Job drawing, mm, ordinate dimensions from the low corner. One solid piece. Coordinates: 2 decimals unless noted, no trailing zeros. Order: outer loops, then holes, each group sorted by start corner. A loop starts at its lowest first (then second) coordinate and runs counter-clockwise, first axis right, second up. Notation, with made-up numbers: M 56.25,-20.75 L 82.25,-20.75 A26 ccw 82.25,8.25 Z; hole C -38.75,54 d3. An arc over 180 degrees is marked long. Write item = value, one per line. Start each with the question number.
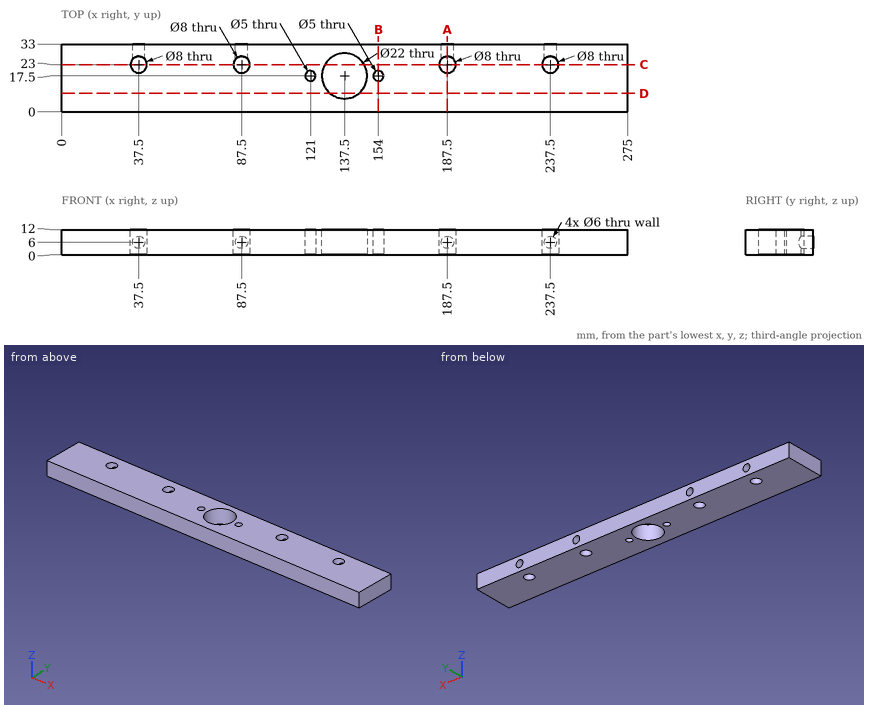
1. Flat gauge pin, fed straight in: pin 1 (5 mm diameter, centred on x = 87.5, z = 6, fed in from +Y). Where does the tip first touch, or does it go through?
2. Slice it at A-A (x = 187.5). Write the cut outline in (y, z).
3. Slice it at C-C (y = 23). Write the cut outline in (x, z).
4. Probe L1, parallel to X at y = 29.75, z = 6; L2, parallel to Y at x = 138.5, z = 1; L3, parallel to Z at x = 38, y = 30. List the from-to ranges inside material, lowest first.
5. Slice it at B-B (x = 154). Write the cut outline in (y, z), plus the area to 3 significant figures.
6. Slice it at D-D (y = 9). Write the cut outline in (x, z).
Calculated:
q1.pin_1 = 19.88
q2.outline = M 0,0 L 19,0 L 19,12 L 0,12 Z; M 27,0 L 33,0 L 33,3 L 27,3 Z; M 27,9 L 33,9 L 33,12 L 27,12 Z
q3.outline = M 0,0 L 33.5,0 L 33.5,12 L 0,12 Z; M 41.5,0 L 83.5,0 L 83.5,12 L 41.5,12 Z; M 91.5,0 L 127.97,0 L 127.97,12 L 91.5,12 Z; M 147.03,0 L 183.5,0 L 183.5,12 L 147.03,12 Z; M 191.5,0 L 233.5,0 L 233.5,12 L 191.5,12 Z; M 241.5,0 L 275,0 L 275,12 L 241.5,12 Z
q4.L1 = 0 to 34.5, 40.5 to 84.5, 90.5 to 184.5, 190.5 to 234.5, 240.5 to 275
q4.L2 = 0 to 6.55, 28.45 to 33
q4.L3 = 0 to 3.04, 8.96 to 12
q5.outline = M 0,0 L 15,0 L 15,12 L 0,12 Z; M 20,0 L 33,0 L 33,12 L 20,12 Z
q5.area = 336 mm²
q6.outline = M 0,0 L 130.52,0 L 130.52,12 L 0,12 Z; M 144.48,0 L 275,0 L 275,12 L 144.48,12 Z
